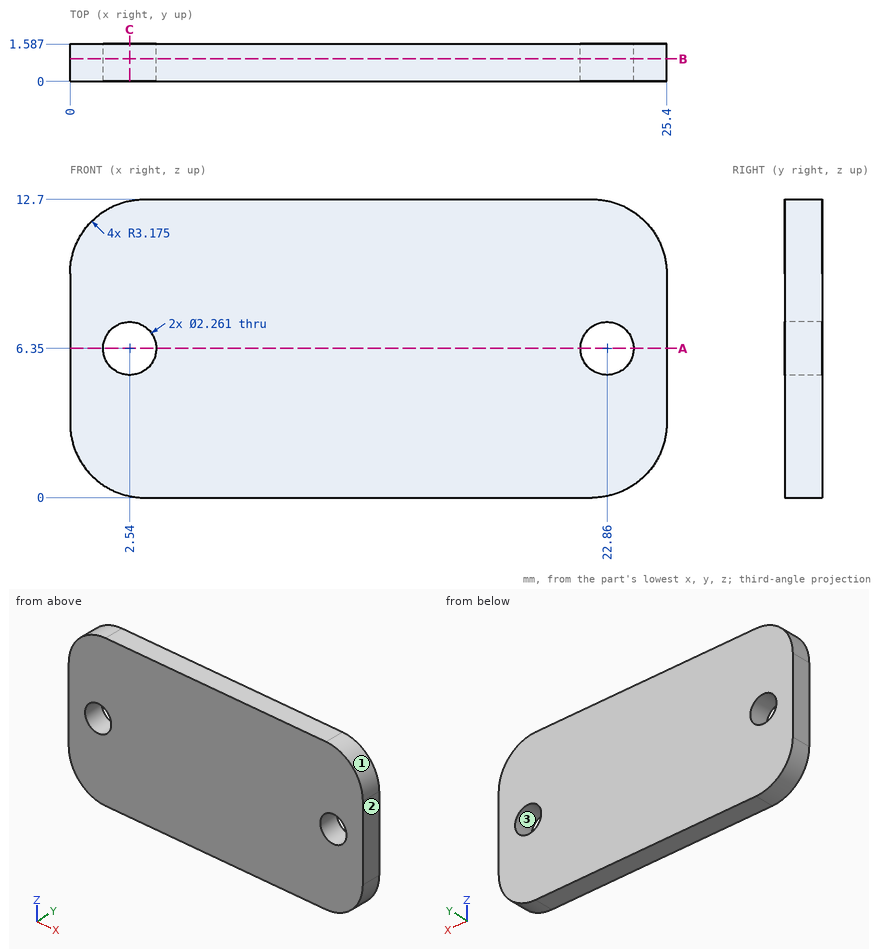
Geometry check sheet. Reference: drawing and pictorial views, mm from the part's lowest x, y, z. Coordinates: 2 decimals unless noted, no trailing zeros. Order: outer loops, then holes, each group sorted by start corner. A loop starts at its lowest first (then second) coordinate and runs counter-clockwise, first axis right, second up. Notation, with made-up numbers: (43.25, -36.75) - (76.25, -36.75) arc R9 ccw to (76.25, -29.75) - close; hole circle Ø4 at (74.25, 57.5). An arc over 180 degrees is marked (long way). Answer in a Markdown table with one row per item. Add a question column.
1) Cross-section at A-A, the plane z = 6.35. Record the cut outline in (x, y).
2) Material ranges on line 1 along X through (y, z) = (1.2, 6.35); line 2 along X through (y, z) = (0.3, 5.5) (1 decimal); line 3 along Z through (x, y) = (22.86, 1.25) (1 decimal), recorded low to high. Write a range as [from, to].
3) Cross-section at C-C, the plane x = 2.54. Record the cut outline in (y, z) (1 decimal).
4) Release check for a two-part mould opening along Z. For the marked faces 1, 2 and 3 record: +Z half, -Z half, draft (parallel to the pull), parting line (faces both ways), or undercut.
5) Cross-section at B-B, the plane y = 0.95. State how many separate pieces and enclosed holes the cut face has, then the cut area to 3 significant figures.
6) Gauge pin test, flat end, axial feed: P1, Ø3, axis at x = 2.54, z = 6.35, coming from the -Y side. Record the tip position at first contact, or that the pin passes through.
Check result:
| question | item | result |
|---|---|---|
| 1 | outline | (0, 0) - (1.41, 0) - (1.41, 1.59) - (0, 1.59) - close; (3.67, 0) - (21.73, 0) - (21.73, 1.59) - (3.67, 1.59) - close; (23.99, 0) - (25.4, 0) - (25.4, 1.59) - (23.99, 1.59) - close |
| 2 | line 1 | x = [0, 1.41], [3.67, 21.73], [23.99, 25.4] |
| 2 | line 2 | x = [0, 1.8], [3.3, 22.1], [23.6, 25.4] |
| 2 | line 3 | z = [0.1, 5.2], [7.5, 12.6] |
| 3 | outline | (0, 0.1) - (1.6, 0.1) - (1.6, 5.2) - (0, 5.2) - close; (0, 7.5) - (1.6, 7.5) - (1.6, 12.6) - (0, 12.6) - close |
| 4 | face 1 | +Z half |
| 4 | face 2 | draft |
| 4 | face 3 | undercut |
| 5 | separate pieces | 1 |
| 5 | enclosed holes | 2 |
| 5 | area | 306 mm² |
| 6 | P1 | stops at y = 0 |
